CAD build for the part. Positions are in the model's coordinates, mm. Face numbers are marked on the shaded views. A direction names the side the tool comes from. Give positions to 0.01 mm unless a question says otherwise; leave off trailing zeros. Write each loop counter-clockwise with the first axis right and the second up, starting at its lowest first coordinate (ties: lowest second). Pieces come first, ordered by that corner, then holes. Notation, with made-up numbers: (-8, 1.25) -> (21, 1.25) arc R21 cw to (21, 31.25) -> close; hole circle Ø1 at (60.5, 50). An arc over 180 degrees is marked (long way). Answer in a Markdown table with one row per item. Add a question column.
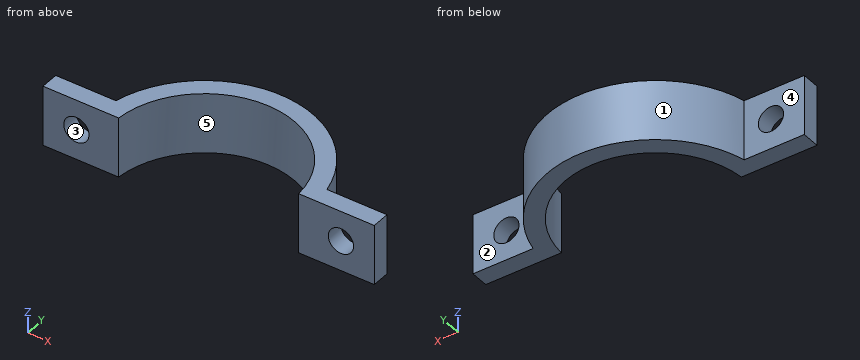
```python
from build123d import *

# Parameters (mm, degrees)
PAD_DEPTH    = 10
SKETCH001_R  = 2.1
POCKET_DEPTH = 134.047902


with BuildPart() as part:
    # Sketch → Pad (new body)
    with BuildSketch(Plane.XY):
        with BuildLine():
            ThreePointArc((14.96663, 0), (0, 14), (-14.96663, 0))
            Line((-27.549929, 0), (-14.96663, 0))
            Line((-27.549929, 3), (-27.549929, 0))
            Line((-17.549929, 3), (-27.549929, 3))
            ThreePointArc((17.549929, 3), (0, 17), (-17.549929, 3))
            Line((27.549929, 3), (17.549929, 3))
            Line((27.549929, 0), (27.549929, 3))
            Line((14.96663, 0), (27.549929, 0))
        make_face()
    extrude(amount=PAD_DEPTH)

    # Sketch001 → Pocket (cut, through all)
    with BuildSketch(Plane.XZ):
        with Locations((-22, 5)):
            Circle(SKETCH001_R)
    pocket = extrude(amount=-POCKET_DEPTH, mode=Mode.SUBTRACT)

    # Mirrored: Pocket across Sketch001 V_Axis
    add(pocket.mirror(Plane(origin=(0, 0, 0), x_dir=(0, -1, 0), z_dir=(1, 0, 0))), mode=Mode.SUBTRACT)


solid = part.part
```
Item 1: Slice it at B-B, the plane z = 5. List the corners of the cut face in (x, y).
Item 2: Mould opens along X. For the marked faces 1, 2 and 3 say: released by +X, released by -X, zero draft, split by the parting line, or undercut.
Item 3: Slice it at A-A, the plane x = -22. List the corners of the cut face in (y, z), then the cut area to 3 significant figures.
Item 4: Slice it at C-C, the plane y = 4.5. List the corners of the cut face in (x, z), then the cut area to 3 significant figures.
Item 5: Slice it at D-D, the plane z = 9. List the corners of the cut face in (x, y).
Item 6: Probe L1, parallel to X at y = 2.75, z = 4; L2, parallel to Y at x = 18.5, z = 7; L3, parallel to X at y = 5, z = 8.75. List the from-to ranges inside material, lowest first. Write a range as from..to.
Item 7: Drop flat-ended pins along their axis: pin 1 Ø5 at (y, z) = (12, 8) entering from -X; pin 2 Ø3 at (y, z) = (5.5, 7) entering from -X; pin 3 Ø6 at (x, y) = (-7, 10) entering from -Z; pin 4 Ø5 at (x, z) = (17, 5) entering from +Y. Give the stop position or say it passes through.
Item 8: Which spindle directions (+Z, -Z, +X, -X, +Y, -Y) get a long thin tool onto all of the face, cutting with end or side? Do the marked faces 4 and 5. Say none if no direction does.
Answer key:
| question | item | result |
|---|---|---|
| 1 | outline | (-27.55, 0) -> (-24.1, 0) -> (-24.1, 3) -> (-27.55, 3) -> close; (-19.9, 0) -> (-14.97, 0) arc R15 cw to (14.97, 0) -> (19.9, 0) -> (19.9, 3) -> (17.55, 3) arc R18 ccw to (-17.55, 3) -> (-19.9, 3) -> close; (24.1, 0) -> (27.55, 0) -> (27.55, 3) -> (24.1, 3) -> close |
| 2 | face 1 | split by the parting line |
| 2 | face 2 | zero draft |
| 2 | face 3 | undercut |
| 3 | outline | (0, 0) -> (3, 0) -> (3, 2.9) -> (0, 2.9) -> close; (0, 7.1) -> (3, 7.1) -> (3, 10) -> (0, 10) -> close |
| 3 | area | 17.4 mm² |
| 4 | outline | (-17.14, 0) -> (-13.96, 0) -> (-13.96, 10) -> (-17.14, 10) -> close; (13.96, 0) -> (17.14, 0) -> (17.14, 10) -> (13.96, 10) -> close |
| 4 | area | 63.7 mm² |
| 5 | outline | (-27.55, 0) -> (-14.97, 0) arc R15 cw to (14.97, 0) -> (27.55, 0) -> (27.55, 3) -> (17.55, 3) arc R18 ccw to (-17.55, 3) -> (-27.55, 3) -> close |
| 6 | L1 | x = -27.55..-23.85, -20.15..-14.52, 14.52..20.15, 23.85..27.55 |
| 6 | L2 | y = 0..3 |
| 6 | L3 | x = -16.97..-13.75, 13.75..16.97 |
| 7 | pin 1 | stops at x = -14.62 |
| 7 | pin 2 | stops at x = -17.29 |
| 7 | pin 3 | stops at z = 0 |
| 7 | pin 4 | stops at y = 9.67 |
| 8 | face 4 | +Z, -Z, -X, +Y |
| 8 | face 5 | +Z, -Z, -Y |
